CAD build for the part. Positions are in the model's coordinates, mm. Give positions to 0.01 mm unless a question says otherwise; leave off trailing zeros. Write each loop counter-clockwise with the first axis right and the second up, starting at its lowest first coordinate (ties: lowest second). Pieces come first, ordered by that corner, then holes. Notation, with made-up numbers: (50, -34.75) -> (92, -34.75) arc R18 cw to (92, -18.75) -> close; hole circle Ø5 at (-0.5, 42.25). An arc over 180 degrees is marked (long way). Answer in a Markdown table with one row per item. Add a question column.
```python
from build123d import *

# Parameters (mm, degrees)
ESTRUSIONE_ESTRUSIONE2_DEPTH      = 150
ESTRUSIONE_ESTRUSIONE2_DEPTH_BACK = 150
ESTRUSIONE_ESTRUSIONE3_DEPTH      = 3.3
ESTRUSIONE_ESTRUSIONE3_DEPTH_BACK = 303.3
SCHIZZO3_W                        = 6.5
SCHIZZO3_H                        = 6.5


with BuildPart() as part:
    # Schizzo2 → Estrusione-Estrusione2 (new, two sides: drawn at the far end of the back side and taken through both)
    with BuildSketch(Plane(origin=(0, 0, 0), x_dir=(1, 0, 0), z_dir=(0, 1, 0)).offset(-ESTRUSIONE_ESTRUSIONE2_DEPTH_BACK)):
        Polygon((-113.15, 106.65), (-113.15, -106.65), (-106.65, -106.65), (-106.65, -113.15), (106.65, -113.15), (106.65, -106.65), (113.15, -106.65), (113.15, 106.65), (106.65, 106.65), (106.65, 113.15), (-106.65, 113.15), (-106.65, 106.65), align=None)
    extrude(amount=ESTRUSIONE_ESTRUSIONE2_DEPTH + ESTRUSIONE_ESTRUSIONE2_DEPTH_BACK)

    # Schizzo3 → Estrusione-Estrusione3 (add, two sides: drawn at the far end of the back side and taken through both)
    with BuildSketch(Plane.XZ.offset(150).offset(-ESTRUSIONE_ESTRUSIONE3_DEPTH_BACK)):
        with Locations((-109.9, 109.9)):
            Rectangle(SCHIZZO3_W, SCHIZZO3_H)
        with Locations((109.9, 109.9)):
            Rectangle(SCHIZZO3_W, SCHIZZO3_H)
        with Locations((109.9, -109.9)):
            Rectangle(SCHIZZO3_W, SCHIZZO3_H)
        with Locations((-109.9, -109.9)):
            Rectangle(SCHIZZO3_W, SCHIZZO3_H)
    extrude(amount=ESTRUSIONE_ESTRUSIONE3_DEPTH + ESTRUSIONE_ESTRUSIONE3_DEPTH_BACK)


solid = part.part
```
Item 1: Slice it at A-A, the plane x = 88.5. List the corners of the cut face in (y, z).
Item 2: Slice it at B-B, the plane z = -35. List the corners of the cut face in (x, y), then the cut area to 3 significant figures.
Item 3: Drop flat-ended pins along their axis: pin 1 Ø8 at (x, z) = (-68, 81.5) entering from +Y; pin 2 Ø3 at (x, z) = (85.5, -33.5) entering from -Y. Give the stop position or say it passes through.
Item 4: Probe L1, parallel to Y at x = 4, z = -51.5. List the from-to ranges inside material, lowest first. Write a range as from..to.
Answer key:
| question | item | result |
|---|---|---|
| 1 | outline | (-150, -113.15) -> (150, -113.15) -> (150, 113.15) -> (-150, 113.15) -> close |
| 2 | outline | (-113.15, -150) -> (113.15, -150) -> (113.15, 150) -> (-113.15, 150) -> close |
| 2 | area | 67,900 mm² |
| 3 | pin 1 | stops at y = 150 |
| 3 | pin 2 | stops at y = -150 |
| 4 | L1 | y = -150..150 |
